Verification items for the finished model (mm, model axes). A direction names the side the tool comes from. Round coordinates to 2 decimals unless told otherwise and drop trailing zeros. Order: outer loops, then holes, each group sorted by start corner. A loop starts at its lowest first (then second) coordinate and runs counter-clockwise, first axis right, second up. Notation, with made-up numbers: M -40,67.25 L -16,67.25 A11 cw -16,82.25 Z; hole C 87.25,45 d6. An arc over 180 degrees is marked long. Return JSON: item names as keys, results as strings. Group by question number.
from build123d import *

# Parameters (mm, degrees)
SKETCH1_R           = 0.9
BOSS_EXTRUDE1_DEPTH = 7
CUT_EXTRUDE1_REACH  = 21.129
SKETCH2_W           = 6
SKETCH2_H           = 3.2
SKETCH3_W           = 11
SKETCH3_H           = 3.7
CUT_EXTRUDE2_DEPTH  = 4
SKETCH6_W           = 4
SKETCH6_H           = 15
BOSS_EXTRUDE2_DEPTH = 0.6275
CUT_EXTRUDE3_REACH  = 24.006


with BuildPart() as part:
    # Sketch1 → Boss-Extrude1 (new body)
    with BuildSketch(Plane(origin=(0, 0, 0), x_dir=(1, 0, 0), z_dir=(0, 1, 0))):
        with BuildLine():
            Line((1.496941475, 0), (13.996941475, 0))
            Line((13.996941475, 0), (13.996941475, -15))
            Line((13.996941475, -15), (9.996941475, -15))
            Line((9.996941475, -15), (9.996941475, -4))
            Line((9.996941475, -4), (1.496941475, -4))
            ThreePointArc((1.496941475, -4), (-0.503058525, -2), (1.496941475, 0))
        make_face()
        with Locations(Location((2.496941475, -2, 0), (0, 0, 270))):
            Circle(SKETCH1_R, mode=Mode.SUBTRACT)
    extrude(amount=BOSS_EXTRUDE1_DEPTH)

    # Sketch2 → Cut-Extrude1 (cut, up to next)
    with BuildSketch(Plane.XY.offset(4), mode=Mode.PRIVATE) as cut_extrude1_sk1:
        with Locations((2.496941475, 3.5)):
            Rectangle(SKETCH2_W, SKETCH2_H)
    cut_extrude1_tool1 = extrude(cut_extrude1_sk1.sketch, amount=-CUT_EXTRUDE1_REACH, mode=Mode.PRIVATE) & part.part
    add(cut_extrude1_tool1.solids().sort_by_distance((2.496941, 3.5, 4))[0], mode=Mode.SUBTRACT)

    # Sketch3 → Cut-Extrude2 (cut)
    with BuildSketch(Plane(origin=(13.996941475, 0, 0), x_dir=(0, 0, -1), z_dir=(1, 0, 0))):
        with Locations((-9.5, 5.15)):
            Rectangle(SKETCH3_W, SKETCH3_H)
    extrude(amount=-CUT_EXTRUDE2_DEPTH, mode=Mode.SUBTRACT)

    # Sketch6 → Boss-Extrude2 (add)
    with BuildSketch(Plane.XZ):
        with Locations((11.996941475, 7.5)):
            Rectangle(SKETCH6_W, SKETCH6_H)
    extrude(amount=BOSS_EXTRUDE2_DEPTH)

    # Sketch4 → Cut-Extrude3 (cut, up to next)
    with BuildSketch(Plane(origin=(13.996941475, 0, 0), x_dir=(0, 0, -1), z_dir=(1, 0, 0)), mode=Mode.PRIVATE) as cut_extrude3_sk1:
        Polygon((-11, -0.6275), (-15, -0.6275), (-15, 1.0225), (-12, 1.0225), (-11, 0.0225), align=None)
    cut_extrude3_tool1 = extrude(cut_extrude3_sk1.sketch, amount=-CUT_EXTRUDE3_REACH, mode=Mode.PRIVATE) & part.part
    add(cut_extrude3_tool1.solids().sort_by_distance((13.996941, 0.157199, 13.136612))[0], mode=Mode.SUBTRACT)


solid = part.part
1. Cross-section at D-D (x = 13). Enter the section's corners in (y, z).
2. Thickness scan on line 1 along X through (y, z) = (0.9, 2); line 2 along X through (y, z) = (1.25, 6.75); line 3 along Y through (x, z) = (3.75, 3). Record the ranges inside material, lowest first. Write a range as from..to.
3. Cross-section at B-B (x = 4.25). Enter the section's corners in (y, z).
4. Draft check along Z on faces 6 (the face through (12, -0.628, 6)), 7 (the face through (1.7, 6.04, 2.42)), 8 (the face through (12.02, 0.53, 11.51)), 9 (the face through (1.7, 0.94, 2.42)). Enter one of: +Z half, -Z half, draft (parallel to the pull), parting line (faces both ways), or undercut.
5. Cross-section at C-C (y = 3). Enter the section's corners in (x, z).
6. Cross-section at A-A (z = 2). Enter the section's corners in (x, y), plus the area to 3 significant figures.
7. Go/stop test with flat-tipped pins: pin 1 (3 mm diameter, centred on x = 6.5, y = 2, fed in from +Z); pin 2 (3.5 mm diameter, centred on x = 11.5, z = 13, fed in from -Y); pin 3 (1.2 mm diameter, centred on x = 11.5, z = 10.5, fed in from +Y). Record where each tip stops, or that it passes through.
8. Access from +Z, -Z, +X, -X, +Y, -Y to the whole of each face (thin tool, end or side, straight path). Record for faces 1 (the face through (7, 7, 2)), 2 (the face through (5, 0, 2)), 3 (the face through (12, 3.3, 10)), 4 (the face through (5.497, 3, 2)), 5 (the face through (12, 1.022, 14)).
Computed:
{
 "1": {"outline": "M -0.63,0 L 7,0 L 7,4 L 3.3,4 L 3.3,15 L 1.02,15 L 1.02,12 L 0.02,11 L -0.63,11 Z"},
 "2": {"line 1": "x = -0.5..1.6, 3.4..14", "line 2": "x = 10..14", "line 3": "y = 0..1.9, 5.1..7"},
 "3": {"outline": "M 0,0 L 1.9,0 L 1.9,4 L 0,4 Z; M 5.1,0 L 7,0 L 7,4 L 5.1,4 Z"},
 "4": {"face 6": "draft", "face 7": "undercut", "face 8": "+Z half", "face 9": "undercut"},
 "5": {"outline": "M 5.5,0 L 14,0 L 14,15 L 10,15 L 10,4 L 5.5,4 Z"},
 "6": {"outline": "M -0.5,0 L 1.6,0 L 1.6,1.9 L -0.5,1.9 Z; M -0.5,5.1 L 1.6,5.1 L 1.6,7 L -0.5,7 Z; M 3.4,0 L 10,0 L 10,-0.63 L 14,-0.63 L 14,7 L 3.4,7 L 3.4,5.1 L 5.5,5.1 L 5.5,1.9 L 3.4,1.9 Z", "area": "78.0 mm²"},
 "7": {"pin 1": "stops at z = 4", "pin 2": "stops at y = 0.27", "pin 3": "stops at y = 3.3"},
 "8": {"face 1": "+Z, -Z, +X, -X, +Y", "face 2": "+Z, -Z, -X, -Y", "face 3": "+Z, +X, -X, +Y", "face 4": "+Z, -Z, -X", "face 5": "+Z, +X, -X, -Y"}
}
